from build123d import *

# Parameters (mm, degrees)
F0_W     = 70
F0_H     = 18.273093
F1_DEPTH = 20
F3_R     = 8.1
F4_DEPTH = 10
F5_R     = 9
F6_DEPTH = 25
F7_R     = 7


with BuildPart() as f1:
    # F0 (on Top) → F1 (new body)
    with BuildSketch(Plane.XY):
        with Locations((0, -0.321428)):
            Rectangle(F0_W, F0_H)
    extrude(amount=F1_DEPTH)

    # F3 (on offset) → F4 (cut)
    with BuildSketch(Plane.XZ.offset(10)):
        with Locations((-24, 10)):
            Circle(F3_R)
        with Locations((24, 10)):
            Circle(F3_R)
    extrude(amount=-F4_DEPTH, mode=Mode.SUBTRACT)

    # F5 (on Top) → F6 (cut)
    with BuildSketch(Plane.XY):
        with Locations((0, 8.815118)):
            Circle(F5_R)
    extrude(amount=F6_DEPTH, mode=Mode.SUBTRACT)

    # F7
    f7_edges = [f1.edges().sort_by_distance(p)[0] for p in [
        (35, 8.815118, 10),
        (-35, 8.815118, 10),
    ]]
    fillet(f7_edges, radius=F7_R)


solid = f1.part
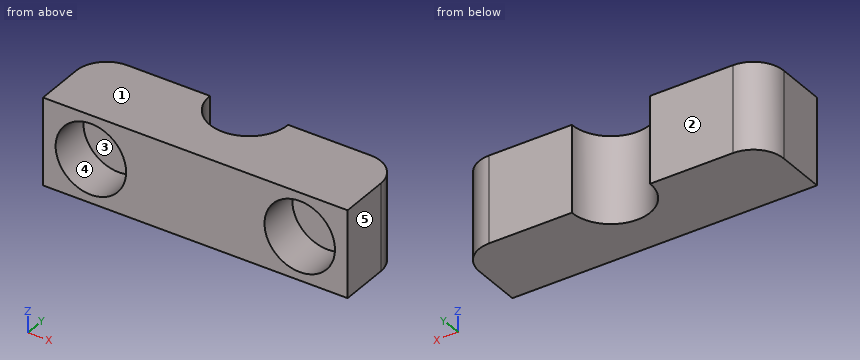
Could you check a few things on this model? Use its own coordinates, in mm. Face numbers are marked on the shaded views. A direction names the side the tool comes from. Give positions to 0.01 mm unless a question says otherwise; leave off trailing zeros. Order: outer loops, then holes, each group sorted by start corner. A loop starts at its lowest first (then second) coordinate and runs counter-clockwise, first axis right, second up. Notation, with made-up numbers: (12.25, 69.25) -> (69.25, 69.25) arc R15 ccw to (69.25, 89.25) -> close; hole circle Ø6 at (-13, 3.5). An arc over 180 degrees is marked (long way). Answer in a Markdown table with one row per item. Add a question column.
Item 1: Please list where these lines run through material, in increasing order: probe 1 along X at (y, z) = (-0.25, 4); probe 2 along Z at (x, y) = (24, -4.75); probe 3 along X at (y, z) = (-6, 3).
Item 2: Imagine slicing it at D-D (y = 7.25). List the corners of the cut face in (x, z) for me, and give its area (3 significant figures).
Item 3: I'm going to push flat-ended pins straight in: P1, Ø6, axis at x = 1.5, z = 3, coming from the +Y side; P2, Ø9.5, axis at x = 24, z = 10, coming from the -Y side; P3, Ø3, axis at x = -7, y = 6, coming from the -Z side; P4, Ø3, axis at y = 3.5, z = 13.5, coming from the -X side. Where does each tip first touch, or does it pass through?
Item 4: For the marked faces 4 and 5, which set-ups out of +Z, -Z, +X, -X, +Y, -Y let a thin tool reach every point of the face, with its end or its side?
Item 5: We'd pull the mould along Z, two halves only. Please class the marked faces 1, 2 and 3: pulls with the +Z half, pulls with the -Z half, needs draft (parallel to the pull), parting line crosses it, or undercut.
Item 6: Imagine slicing it at B-B (y = 2.5). List the corners of the cut face in (x, z) for me, and give its area (3 significant figures).
Item 7: Imagine slicing it at C-C (z = 10). List the corners of the cut face in (x, y) for me, and give its area (3 significant figures).
Item 8: Imagine slicing it at A-A (x = 24). List the corners of the cut face in (y, z) for me, and give its area (3 significant figures).
Result:
| question | item | result |
|---|---|---|
| 1 | probe 1 | -35 to -29.44, -18.56 to 18.56, 29.44 to 35 |
| 1 | probe 2 | 0 to 1.9, 18.1 to 20 |
| 1 | probe 3 | -35 to -28.08, -19.92 to 19.92, 28.08 to 35 |
| 2 | outline | (-32.41, 0) -> (-8.86, 0) -> (-8.86, 20) -> (-32.41, 20) -> close; (8.86, 0) -> (32.41, 0) -> (32.41, 20) -> (8.86, 20) -> close |
| 2 | area | 942 mm2 |
| 3 | P1 | y = 1.02 |
| 3 | P2 | y = 0 |
| 3 | P3 | z = 0 |
| 3 | P4 | x = -35 |
| 4 | face 4 | -Y |
| 4 | face 5 | +Z, -Z, +X, +Y, -Y |
| 5 | face 1 | pulls with the +Z half |
| 5 | face 2 | needs draft |
| 5 | face 3 | undercut |
| 6 | outline | (-34.97, 0) -> (-6.41, 0) -> (-6.41, 20) -> (-34.97, 20) -> close; (6.41, 0) -> (34.97, 0) -> (34.97, 20) -> (6.41, 20) -> close |
| 6 | area | 1,140 mm2 |
| 7 | outline | (-35, -9.46) -> (-32.1, -9.46) -> (-32.1, 0) -> (-15.9, 0) -> (-15.9, -9.46) -> (15.9, -9.46) -> (15.9, 0) -> (32.1, 0) -> (32.1, -9.46) -> (35, -9.46) -> (35, 1.82) arc R7 ccw to (28, 8.82) -> (9, 8.82) arc R9 cw to (-9, 8.82) -> (-28, 8.82) arc R7 ccw to (-35, 1.82) -> close |
| 7 | area | 824 mm2 |
| 8 | outline | (-9.46, 0) -> (8.82, 0) -> (8.82, 20) -> (-9.46, 20) -> (-9.46, 18.1) -> (0, 18.1) -> (0, 1.9) -> (-9.46, 1.9) -> close |
| 8 | area | 212 mm2 |
